```python
from build123d import *

# Parameters (mm, degrees)
BOSS_EXTRUDE1_DEPTH = 6.35
BOSS_EXTRUDE2_DEPTH = 6.35


with BuildPart() as part:
    # Sketch1 → Boss-Extrude1 (new body)
    with BuildSketch(Plane.XY):
        Polygon((12.5, 72.3975), (18.85, 72.3975), (18.85, 120.6625), (7.5, 120.6625), (7.5, 127.0125), (2.5, 127.0125), (2.5, 120.6625), (-2.5, 120.6625), (-2.5, 127.0125), (-7.5, 127.0125), (-7.5, 120.6625), (-39.5, 120.6625), (-39.5, -80.6625), (-27.5, -80.6625), (-27.5, -120.6625), (-7.5, -120.6625), (-7.5, -127.0125), (-2.5, -127.0125), (-2.5, -120.6625), (2.5, -120.6625), (2.5, -127.0125), (7.5, -127.0125), (7.5, -120.6625), (18.85, -120.6625), (18.85, -72.3975), (12.5, -72.3975), (12.5, -24.1325), (18.85, -24.1325), (18.85, 24.1325), (12.5, 24.1325), align=None)
    extrude(amount=BOSS_EXTRUDE1_DEPTH)

    # Sketch3 → Boss-Extrude2 (add)
    with BuildSketch(Plane.XY.offset(6.35)):
        Polygon((-27.54064, -80.70314), (-27.54064, -120.70314), (-7.54064, -120.70314), (-7.54064, -127.05314), (-2.45936, -127.05314), (-2.45936, -120.70314), (2.45936, -120.70314), (2.45936, -127.05314), (7.54064, -127.05314), (7.54064, -120.70314), (18.89064, -120.70314), (18.89064, -72.35686), (12.54064, -72.35686), (12.54064, -24.17314), (18.89064, -24.17314), (18.89064, 24.17314), (12.54064, 24.17314), (12.54064, 72.35686), (18.89064, 72.35686), (18.89064, 120.70314), (7.54064, 120.70314), (7.54064, 127.05314), (2.45936, 127.05314), (2.45936, 120.70314), (-2.45936, 120.70314), (-2.45936, 127.05314), (-7.54064, 127.05314), (-7.54064, 120.70314), (-39.54064, 120.70314), (-39.54064, -80.70314), align=None)
    extrude(amount=-BOSS_EXTRUDE2_DEPTH)


solid = part.part
```
CAD build for the part. Positions are in the model's coordinates, mm. A direction names the side the tool comes from. Coordinates: 2 decimals unless noted, no trailing zeros. Order: outer loops, then holes, each group sorted by start corner. A loop starts at its lowest first (then second) coordinate and runs counter-clockwise, first axis right, second up. Notation, with made-up numbers: (66, -31.5) - (85, -31.5) arc R27 cw to (85, -13.5) - close; hole circle Ø5 at (5.25, 72). An arc over 180 degrees is marked (long way). Use a Markdown table: item, result. Add a question column.
(1) Saw through at B-B (x = -18). Give the cut face in (y, z), then the cut area to 3 significant figures.
(2) Which spindle directions (+Z, -Z, +X, -X, +Y, -Y) get a long thin tool onto all of the face, cutting with end or side? Do faces 4 (the face through (7.541, -124, 3)), 5 (the face through (-23, 120.703, 3)), 6 (the face through (16, -72.357, 3)), 7 (the face through (7.541, 124, 3)). Say none if no direction does.
(3) Saw through at C-C (y = -35). Give the cut face in (x, z), then the cut area to 3 significant figures.
(4) Pull direction Y, two halves, no side cores. Call faces 1 (the face through (-34, -80.703, 3)), 2 (the face through (12.541, 48, 3)), 3 (the face through (-27.541, -100, 3)): +Y half, -Y half, draft (parallel to the pull), parting line (faces both ways), or undercut.
(5) Flat gauge pins, fed straight in: pin 1 (2.5 mm diameter, centred on x = 0.5, z = 4.5, fed in from +Y); pin 2 (3 mm diameter, centred on y = -106.5, z = 4, fed in from -X); pin 3 (1 mm diameter, centred on x = 0, y = -99, fed in from -Z); pin 4 (1.9 mm diameter, centred on x = 16, z = 4, fed in from -Y). Where does each tip first touch, or does it go through?
(6) Drill centre lines: line 1 along Y through (x, z) = (14, 5.75); line 2 along Y through (x, z) = (1.5, 2); line 3 along Y through (x, z) = (-35.5, 5.75). Where is each one in solid material? Low to high. Write a range as [from, to].
Solved:
| question | item | result |
|---|---|---|
| 1 | outline | (-120.7, 0) - (120.7, 0) - (120.7, 6.35) - (-120.7, 6.35) - close |
| 1 | area | 1,530 mm² |
| 2 | face 4 | +Z, -Z, +X, -Y |
| 2 | face 5 | +Z, -Z, -X, +Y |
| 2 | face 6 | +Z, -Z, +X |
| 2 | face 7 | +Z, -Z, +X, +Y |
| 3 | outline | (-39.54, 0) - (12.54, 0) - (12.54, 6.35) - (-39.54, 6.35) - close |
| 3 | area | 331 mm² |
| 4 | face 1 | -Y half |
| 4 | face 2 | undercut |
| 4 | face 3 | draft |
| 5 | pin 1 | stops at y = 120.7 |
| 5 | pin 2 | stops at x = -27.54 |
| 5 | pin 3 | stops at z = 0 |
| 5 | pin 4 | stops at y = -120.7 |
| 6 | line 1 | y = [-120.7, -72.36], [-24.17, 24.17], [72.36, 120.7] |
| 6 | line 2 | y = [-120.7, 120.7] |
| 6 | line 3 | y = [-80.7, 120.7] |
